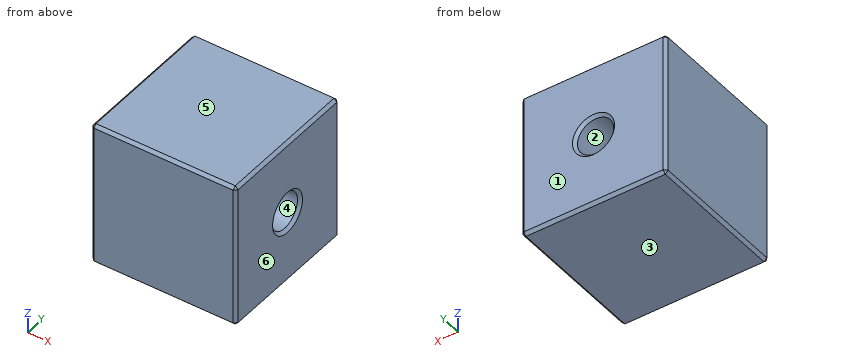
```python
from build123d import *

# Parameters (mm, degrees)
SKETCH_1_W                   = 10
SKETCH_1_H                   = 10
EXTRUDE_1_DEPTH              = 5
HOLE_START                   = 1.25
HOLE_WIZARD_M3_2_OUTLINE_R   = 1.25
HOLE_WIZARD_M3_2_DEPTH       = 3.75
HOLE_START_2                 = -1.2500001
HOLE_WIZARD_M3_2_2_OUTLINE_R = 1.25
HOLE_WIZARD_M3_2_2_DEPTH     = 2.5000001
HOLE_WIZARD_M3_2_3_OUTLINE_W = 6
HOLE_WIZARD_M3_2_3_OUTLINE_H = 6
HOLE_WIZARD_M3_2_3_DEPTH     = 3
HOLE_WIZARD_M3_3_REACH       = 14.247
HOLE_WIZARD_M3_3_BORE_R      = 1.25
CHAMFER_1_SIZE               = 0.2


with BuildPart() as part:
    # 草图1 → 凸台-拉伸1 (new, symmetric)
    with BuildSketch(Plane(origin=(0, 0, 0), x_dir=(1, 0, 0), z_dir=(0, 1, 0))):
        Rectangle(SKETCH_1_W, SKETCH_1_H)
    extrude(amount=EXTRUDE_1_DEPTH, both=True)

    # M3 螺纹孔2: read off the stored shape, not the designer's step
    # M3 螺纹孔2 outline → M3 螺纹孔2 (cut)
    with BuildSketch(Plane(origin=(0, 0, 0), x_dir=(1, 0, 0), z_dir=(0, 1, 0)).offset(HOLE_START)):
        Circle(HOLE_WIZARD_M3_2_OUTLINE_R)
    extrude(amount=HOLE_WIZARD_M3_2_DEPTH, mode=Mode.SUBTRACT)

    # Hole Wizard M3 _2 2 outline → Hole Wizard M3 _2 2 (cut)
    with BuildSketch(Plane(origin=(0, 0, 0), x_dir=(1, 0, 0), z_dir=(0, 1, 0)).offset(HOLE_START_2)):
        Circle(HOLE_WIZARD_M3_2_2_OUTLINE_R)
    extrude(amount=HOLE_WIZARD_M3_2_2_DEPTH, mode=Mode.SUBTRACT)

    # Hole Wizard M3 _2 3 outline → Hole Wizard M3 _2 3 (add)
    with BuildSketch(Plane(origin=(0, 0, 0), x_dir=(0.707106781186548, 0.707106781186547, 0), z_dir=(0.707106781186547, -0.707106781186548, 0))):
        Rectangle(HOLE_WIZARD_M3_2_3_OUTLINE_W, HOLE_WIZARD_M3_2_3_OUTLINE_H)
    extrude(amount=HOLE_WIZARD_M3_2_3_DEPTH)

    # M3 螺纹孔3 bore → M3 螺纹孔3 (cut, up to next)
    with BuildSketch(Plane(origin=(5, 0, 0), x_dir=(0, 0, -1), z_dir=(1, 0, 0)), mode=Mode.PRIVATE) as hole_wizard_m3_3_sk1:
        Circle(HOLE_WIZARD_M3_3_BORE_R)
    hole_wizard_m3_3_tool1 = extrude(hole_wizard_m3_3_sk1.sketch, amount=-HOLE_WIZARD_M3_3_REACH, mode=Mode.PRIVATE) & part.part
    add(hole_wizard_m3_3_tool1.solids().sort_by_distance((5, 0, 0))[0], mode=Mode.SUBTRACT)

    # 倒角1
    chamfer_1_edges = [part.edges().sort_by_distance(p)[0] for p in [
        (-5, 5, 0),
        (-1.25, 5, 0),
        (0, 5, 5),
        (5, 0, 1.25),
        (5, 5, 0),
        (0, -5, 5),
        (-5, -5, 0),
        (0, -5, -5),
        (5, -5, 0),
        (5, 0, 5),
        (-5, 0, 5),
        (-5, 0, -5),
        (5, 0, -5),
        (0, 5, -5),
    ]]
    chamfer(chamfer_1_edges, length=CHAMFER_1_SIZE)


solid = part.part
```
Work out the finished part from the listing and answer in its coordinate system (mm). Face numbers are marked on the shaded views. A direction names the side the tool comes from. Give positions to 0.01 mm unless a question says otherwise; leave off trailing zeros. Loops run counter-clockwise (first coordinate to the right, second up) from the corner with the lowest first, then second, coordinate; pieces in that order, holes last. Notation, with made-up numbers: M -39.5,27 L -7.5,27 A14 cw -7.5,53 Z; hole C 72.5,-7 d3. An arc over 180 degrees is marked long. One line per item, written item: value. Start each with the question number.
1. Find section D-D (y = 0). Give the vertices of the cut face in (x, z), and give its area (3 significant figures).
2. Each of these flat-tipped pins is pushed along its axis until it touches: P1, Ø1.5, axis at y = 0, z = 0, coming from the +X side; P2, Ø1.5, axis at x = 0, z = 0, coming from the +Y side. Where does it stop, or does it pass through?
3. Find section A-A (z = 0). Give the vertices of the cut face in (x, y), and give its area (3 significant figures).
4. Determine the mould class of the marked faces 3, 4, 5 and 6 for opening direction Z: released by +Z, released by -Z, zero draft, split by the parting line, or undercut.
5. Which of the six approach directions +Z, -Z, +X, -X, +Y, -Y give full straight-line access (tool end or side, diameter ignored) to the marked faces 1 and 2?
6. Find the intervals of material crossed by probe 1 along Y at (x, z) = (3, 0), in increasing order.
7. Find section B-B (x = 2.25). Give the vertices of the cut face in (y, z), and give its area (3 significant figures).
Reported:
1. outline: M -5,-4.8 L -4.8,-5 L 4.8,-5 L 5,-4.8 L 5,-1.45 L 4.8,-1.25 L 0,-1.25 A1.25 cw 0,1.25 L 4.8,1.25 L 5,1.45 L 5,4.8 L 4.8,5 L -4.8,5 L -5,4.8 Z
1. area: 84.9 mm²
2. P1: stops at x = -1
2. P2: stops at y = -1
3. outline: M -5,-4.8 L -4.8,-5 L 4.8,-5 L 5,-4.8 L 5,-1.45 L 4.8,-1.25 L -1.25,-1.25 L -1.25,4.8 L -1.45,5 L -4.8,5 L -5,4.8 Z; M 1.25,1.25 L 4.8,1.25 L 5,1.45 L 5,4.8 L 4.8,5 L 1.45,5 L 1.25,4.8 Z
3. area: 74.8 mm²
4. face 3: released by -Z
4. face 4: undercut
4. face 5: released by +Z
4. face 6: zero draft
5. face 1: +Z, -Z, +X, -X, +Y
5. face 2: +Y
6. probe 1: y = -5 to -1.25, 1.25 to 5
7. outline: M -5,-4.8 L -4.8,-5 L 4.8,-5 L 5,-4.8 L 5,4.8 L 4.8,5 L -4.8,5 L -5,4.8 Z; hole C 0,0 d2.5
7. area: 95.0 mm²
